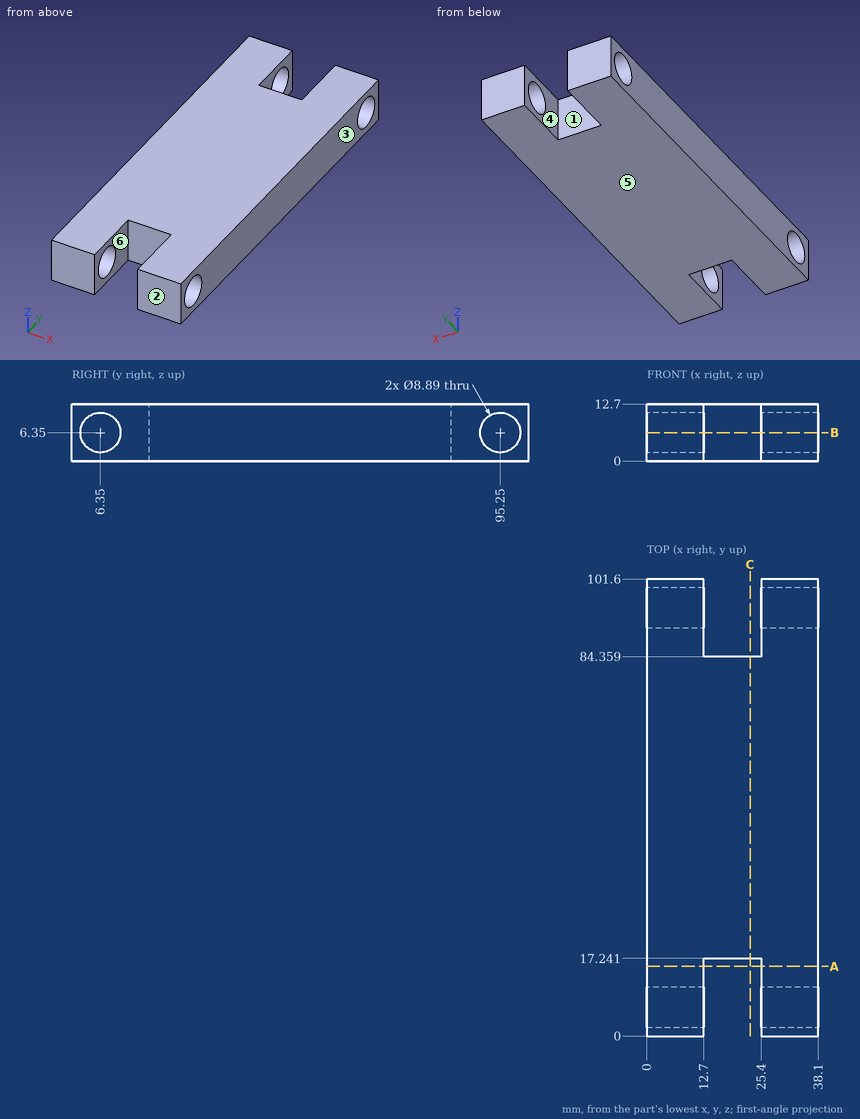
Geometry: see drawing. Coordinates: mm, zero at the bounding-box minimum. A direction names the side the tool comes from. Coordinates: 2 decimals unless noted, no trailing zeros. Loops run counter-clockwise (first coordinate to the right, second up) from the corner with the lowest first, then second, coordinate; pieces in that order, holes last. Notation, with made-up numbers: M 54,68.5 L 101,68.5 A11 ccw 101,88.5 Z; hole C 38.25,26.25 d11. An arc over 180 degrees is marked long. Answer in a Markdown table with one row per item.
Q1. Section C-C on x = 23. Return the cut outline in (y, z).
Answers below:
| item | result |
|---|---|
| outline | M 17.24,0 L 84.36,0 L 84.36,12.7 L 17.24,12.7 Z |
Q2. Section B-B on z = 6.35. Return the cut outline in (x, y) (1 decimal), plus the area to 3 significant figures.
Answers below:
| item | result |
|---|---|
| outline | M 0,0 L 12.7,0 L 12.7,1.9 L 0,1.9 Z; M 0,10.8 L 12.7,10.8 L 12.7,17.2 L 25.4,17.2 L 25.4,10.8 L 38.1,10.8 L 38.1,90.8 L 25.4,90.8 L 25.4,84.4 L 12.7,84.4 L 12.7,90.8 L 0,90.8 Z; M 0,99.7 L 12.7,99.7 L 12.7,101.6 L 0,101.6 Z; M 25.4,0 L 38.1,0 L 38.1,1.9 L 25.4,1.9 Z; M 25.4,99.7 L 38.1,99.7 L 38.1,101.6 L 25.4,101.6 Z |
| area | 2,980 mm^2 |
Q3. Set-up query: the marked faces 4, 5 and 6. Return all of +Z, -Z, +X, -X, +Y, -Y with unobstructed straight access to the full face (end or side cutting, diameter ignored); none if empty.
Answers below:
| item | result |
|---|---|
| face 4 | +Z, -Z, +Y |
| face 5 | -Z, +X, -X, +Y, -Y |
| face 6 | +Z, -Z, -Y |
Q4. Section A-A on y = 15.5. Return the cut outline in (x, z).
Answers below:
| item | result |
|---|---|
| outline | M 0,0 L 12.7,0 L 12.7,12.7 L 0,12.7 Z; M 25.4,0 L 38.1,0 L 38.1,12.7 L 25.4,12.7 Z |
Q5. Ray query, probe 1 along Z at (x, y) = (6, 95.25) (1 decimal); probe 2 along X at (y, z) = (95, 1.25); probe 3 along Y at (x, z) = (34.5, 4.75). Return the intervals inside material, ascending. Write a range as from..to.
Answers below:
| item | result |
|---|---|
| probe 1 | z = 0..1.9, 10.8..12.7 |
| probe 2 | x = 0..12.7, 25.4..38.1 |
| probe 3 | y = 0..2.2, 10.5..91.1, 99.4..101.6 |
Q6. First-contact query: pin 1 (4 mm diameter, centred on y = 63, z = 9, fed in from -X); pin 2 (4 mm diameter, centred on x = 16.5, z = 5, fed in from -Y). Flat tips, straight axial feed; report the tip coordinate or a pass-through.
Answers below:
| item | result |
|---|---|
| pin 1 | stops at x = 0 |
| pin 2 | stops at y = 17.24 |
Q7. Draft query along X for the marked faces 1, 2 and 3. Return one class per face: pulls with the +X half, pulls with the -X half, needs draft (parallel to the pull), parting line crosses it, or undercut.
Answers below:
| item | result |
|---|---|
| face 1 | undercut |
| face 2 | needs draft |
| face 3 | pulls with the +X half |
